Geometry: final body of the model. Coordinates: model frame, mm. Face numbers are marked on the shaded views. A direction names the side the tool comes from. Round coordinates to 2 decimals unless told otherwise and drop trailing zeros. Loops run counter-clockwise (first coordinate to the right, second up) from the corner with the lowest first, then second, coordinate; pieces in that order, holes last. Notation, with made-up numbers: (30, 77) - (51, 77) arc R34 ccw to (51, 111) - close; hole circle Ø3 at (-35.75, 67.25). An arc over 180 degrees is marked (long way). Return JSON: item names as keys, results as strings. Group by question number.
1. Set-up query: the marked faces 1 and 2. Return all of +Z, -Z, +X, -X, +Y, -Y with unobstructed straight access to the full face (end or side cutting, diameter ignored); none if empty.
2. Material intervals for probe 1 along X at (y, z) = (0.5, 0.5) (3 decimals); probe 2 along Y at (x, z) = (4.75, -2.05); probe 3 along Z at (x, y) = (5, 0), sorted ascending.
3. First-contact query: pin 1 Ø1 at (x, z) = (0.5, 0.5) entering from +Y; pin 2 Ø1.2 at (x, z) = (0.5, -2) entering from +Y. Flat tips, straight axial feed; report the tip coordinate or a pass-through.
4. Section D-D on z = 0. Return loops of the section in (x, y) (3 decimals).
5. Section B-B on y = 0.5. Return loops of the section in (x, z) (3 decimals).
6. Section C-C on x = 2.54. Return loops of the section in (y, z).
7. Section A-A on z = -3. Return loops of the section in (x, y) (3 decimals).
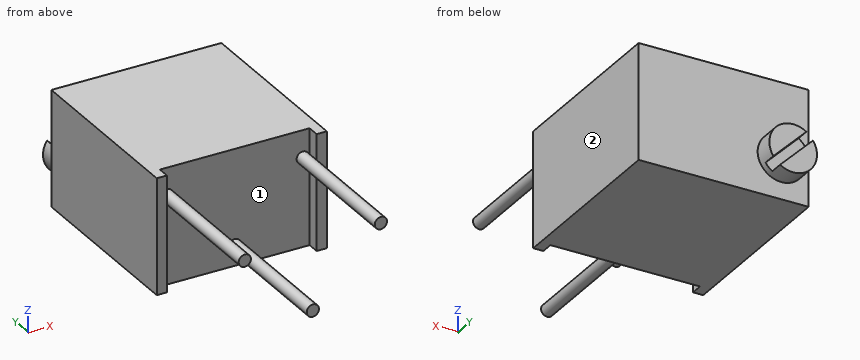
from build123d import *

# Parameters (mm, degrees)
SKETCH3_W               = 6.35
SKETCH3_H               = 6.858
BASE_EXTRUDE_DEPTH      = 1.016
BASE_EXTRUDE_DEPTH_BACK = 3.302
SKETCH4_W               = 5.588
SKETCH4_H               = 0.4572
CUT_EXTRUDE1_DEPTH      = 5.318
SKETCH5_R               = 0.889
BOSS_EXTRUDE1_DEPTH     = 0.762
CUT_EXTRUDE2_DEPTH      = 0.508
SKETCH7_R               = 0.2286
BOSS_EXTRUDE2_DEPTH     = 5.08


with BuildPart() as part:
    # Sketch3 → Base-Extrude (new body, two sides)
    with BuildSketch(Plane.XY) as base_extrude_sk:
        with Locations((2.54, 3.683)):
            Rectangle(SKETCH3_W, SKETCH3_H)
    extrude(amount=BASE_EXTRUDE_DEPTH)
    extrude(base_extrude_sk.sketch, amount=-BASE_EXTRUDE_DEPTH_BACK)

    # Sketch4 → Cut-Extrude1 (cut, through all)
    with BuildSketch(Plane.XY.offset(1.016)):
        with Locations((2.54, 0.4826)):
            Rectangle(SKETCH4_W, SKETCH4_H)
    extrude(amount=-CUT_EXTRUDE1_DEPTH, mode=Mode.SUBTRACT)

    # Sketch5 → Boss-Extrude1 (add)
    with BuildSketch(Plane(origin=(0, 7.112, 0), x_dir=(-1, 0, 0), z_dir=(0, 1, 0))):
        with Locations((-0.381, -1.778)):
            Circle(SKETCH5_R)
    extrude(amount=BOSS_EXTRUDE1_DEPTH)

    # Sketch6 → Cut-Extrude2 (cut)
    with BuildSketch(Plane(origin=(0, 7.874, 0), x_dir=(-1, 0, 0), z_dir=(0, 1, 0))):
        Polygon((-1.153302026, -2.801749198), (0.642749198, -1.005697974), (0.391302026, -0.754250802), (-1.404749198, -2.550302026), align=None)
    extrude(amount=-CUT_EXTRUDE2_DEPTH, mode=Mode.SUBTRACT)

    # Sketch7 → Boss-Extrude2 (add)
    with BuildSketch(Plane.XZ.offset(-0.7112)):
        Circle(SKETCH7_R)
        with Locations((5.08, 0)):
            Circle(SKETCH7_R)
        with Locations((2.54, -2.54)):
            Circle(SKETCH7_R)
    extrude(amount=BOSS_EXTRUDE2_DEPTH)


solid = part.part
Taken from the geometry:
{
 "1": {"face 1": "-Y", "face 2": "+Z, -Z, +X, +Y, -Y"},
 "2": {"probe 1": "-0.635 to -0.254, 5.334 to 5.715", "probe 2": "0.71 to 7.11", "probe 3": "-0.21 to 0.21"},
 "3": {"pin 1": "y = 7.11", "pin 2": "y = 7.87"},
 "4": {"outline": "(-0.635, 0.254) - (-0.254, 0.254) - (-0.254, 0.711) - (-0.229, 0.711) - (-0.229, -4.369) - (0.229, -4.369) - (0.229, 0.711) - (4.851, 0.711) - (4.851, -4.369) - (5.309, -4.369) - (5.309, 0.711) - (5.334, 0.711) - (5.334, 0.254) - (5.715, 0.254) - (5.715, 7.112) - (-0.635, 7.112) - close"},
 "5": {"outline": "(-0.635, -3.302) - (-0.254, -3.302) - (-0.254, 1.016) - (-0.635, 1.016) - close; circle Ø0.457 at (0, 0); circle Ø0.457 at (2.54, -2.54); circle Ø0.457 at (5.08, 0); (5.334, -3.302) - (5.715, -3.302) - (5.715, 1.016) - (5.334, 1.016) - close"},
 "6": {"outline": "(-4.37, -2.77) - (0.71, -2.77) - (0.71, -3.3) - (7.11, -3.3) - (7.11, 1.02) - (0.71, 1.02) - (0.71, -2.31) - (-4.37, -2.31) - close"},
 "7": {"outline": "(-0.635, 0.254) - (-0.254, 0.254) - (-0.254, 0.711) - (5.334, 0.711) - (5.334, 0.254) - (5.715, 0.254) - (5.715, 7.112) - (-0.635, 7.112) - close"}
}
